Study the drawing (mm; zero at the part's minimum x, y, z) and answer. Coordinates: 2 decimals unless noted, no trailing zeros. Loops run counter-clockwise (first coordinate to the right, second up) from the corner with the lowest first, then second, coordinate; pieces in that order, holes last. Notation, with made-up numbers: (-7.5, -1) -> (-0.5, -1) arc R12 cw to (-0.5, 17) -> close; hole circle Ø9 at (-7, 67). An arc over 180 degrees is marked (long way). Answer as a JSON object with one key per item and string values. Group by question number.
Q1. Straight lines are drawn through the part: line 1 along X through (y, z) = (3.1, 12.7); line 2 along Z through (x, y) = (16, 1.45); line 3 along X through (y, z) = (3, 71.5) (1 decimal). For each, find the intervals that lie inside material, in ascending order. Write a range as [from, to].
Q2. The part is cut by section A-A on z = 12.7. Write down the section's boundary in (x, y), and give its area (3 significant figures).
Q3. The part is cut by section B-B on y = 3.65. State how many separate pieces and enclosed holes the cut face has, and give its area (3 significant figures).
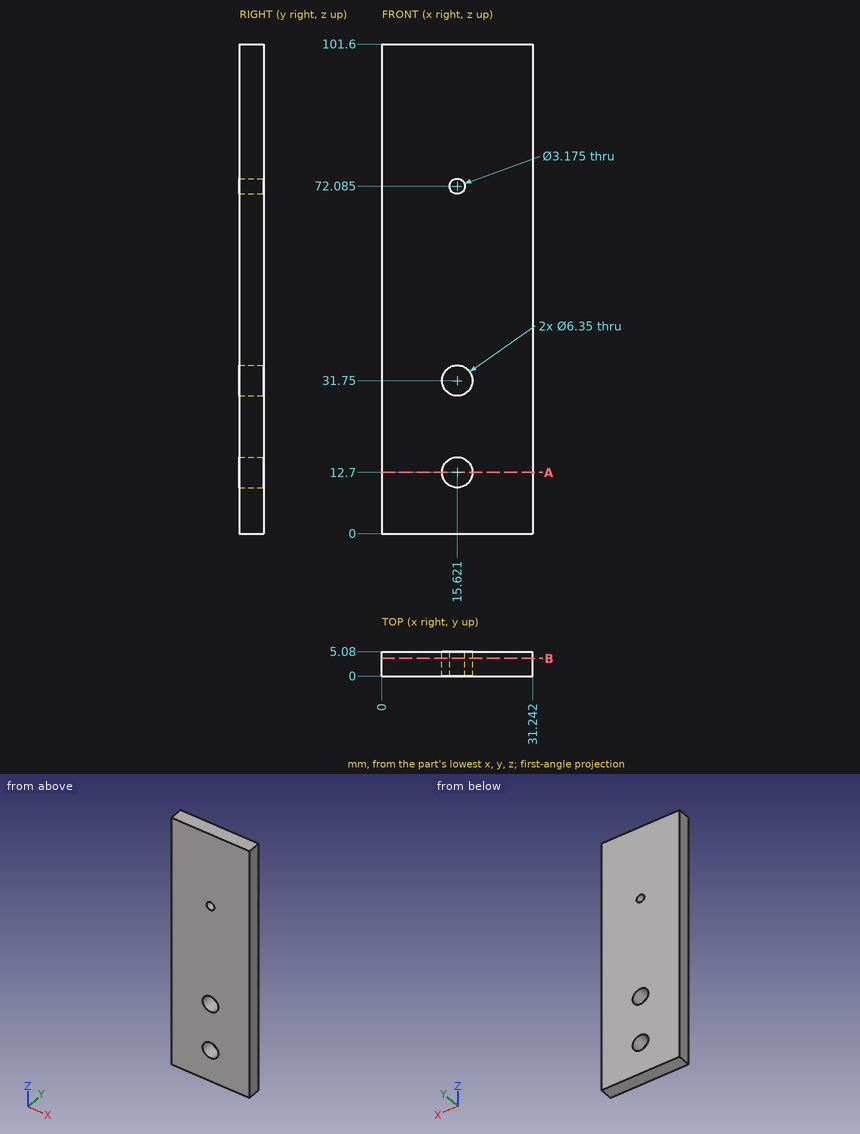
Final values:
{
 "1": {"line 1": "x = [0, 12.45], [18.8, 31.24]", "line 2": "z = [0, 9.55], [15.85, 28.6], [34.9, 70.54], [73.63, 101.6]", "line 3": "x = [0, 14.1], [17.1, 31.2]"},
 "2": {"outline": "(0, 0) -> (12.45, 0) -> (12.45, 5.08) -> (0, 5.08) -> close; (18.8, 0) -> (31.24, 0) -> (31.24, 5.08) -> (18.8, 5.08) -> close", "area": "126 mm2"},
 "3": {"separate pieces": "1", "enclosed holes": "3", "area": "3,100 mm2"}
}
